from build123d import *

# Parameters (mm, degrees)
F1_DEPTH       = 3
F2_DEPTH       = 5.8
F3_D           = 3.3
F3_CSINK_D     = 6.72
F3_CSINK_ANGLE = 90


with BuildPart() as f1:
    # F0 (on Top) → F1 (new body)
    with BuildSketch(Plane.XY):
        with BuildLine():
            ThreePointArc((-3, 0), (0, 3), (3, 0))
            Line((3, 0), (45, 0))
            Line((45, 0), (45, 15))
            Line((45, 15), (-45, 15))
            Line((-45, 15), (-45, 0))
            Line((-45, 0), (-3, 0))
        make_face()
        with BuildLine():
            Line((45, 0), (3, 0))
            ThreePointArc((3, 0), (0, -3), (-3, 0))
            Line((-3, 0), (-45, 0))
            Line((-45, 0), (-45, -15))
            Line((-45, -15), (45, -15))
            Line((45, -15), (45, 0))
        make_face()
    extrude(amount=F1_DEPTH)

    # F0 (on Top) → F2 (join)
    with BuildSketch(Plane.XY):
        with BuildLine():
            Line((-3, 0), (3, 0))
            ThreePointArc((3, 0), (0, 3), (-3, 0))
        make_face()
        with BuildLine():
            ThreePointArc((-3, 0), (0, -3), (3, 0))
            Line((3, 0), (-3, 0))
        make_face()
    extrude(amount=F2_DEPTH)

    # F3 (through all)
    with Locations(Plane(origin=(0, 0, 0), x_dir=(1, 0, 0), z_dir=(0, 0, -1))):
        with Locations((-37, 0), (37, 0)):
            CounterSinkHole(F3_D / 2, F3_CSINK_D / 2, counter_sink_angle=F3_CSINK_ANGLE)


solid = f1.part
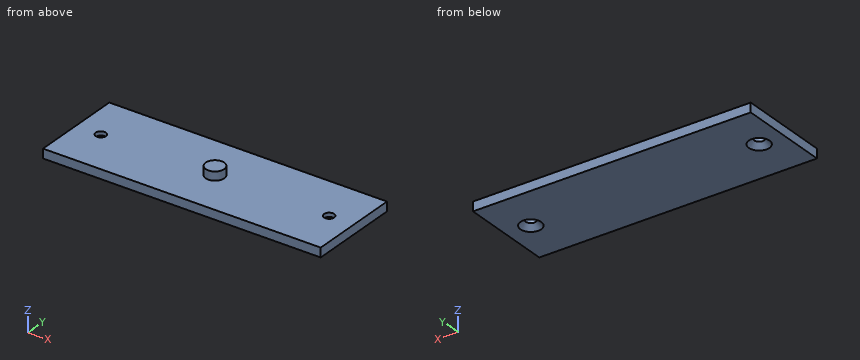
Design review of the part built by this model. Coordinates are the model's own, in mm. Round coordinates to 2 decimals unless told otherwise and drop trailing zeros. Write each loop counter-clockwise with the first axis right and the second up, starting at its lowest first coordinate (ties: lowest second). Pieces come first, ordered by that corner, then holes. Notation, with made-up numbers: (47.25, 72.25) - (65.25, 72.25) arc R6 cw to (65.25, 79.25) - close; hole circle Ø7 at (14, 64.5). An arc over 180 degrees is marked (long way). Use a Markdown table: item, result. Add a question column.
1. We need section B-B (x = 37). State the section outline as (y, z) points, then the cut area to 3 significant figures.
2. We need section D-D (z = 4.55). State the section outline as (x, y) points, then the cut area to 3 significant figures.
3. Clearance check with a flat-ended pin moving along its axis: pin 1 (15 mm diameter, centred on x = -20.5, y = 1.5, fed in from +Z). State where the tip first meets the part, or that it passes through.
4. We need section A-A (y = 0). State the section outline as (x, z) points, then the cut area to 3 significant figures.
5. We need section C-C (x = 0). State the section outline as (y, z) points.
6. Wall thickness on probe 1 along Y at (x, z) = (37, 2.4); probe 2 along Z at (x, y) = (-22.5, 5.75); probe 3 along X at (y, z) = (2.5, 5.15): over which ranges is each line inside the solid? List them lowest first.
Output:
| question | item | result |
|---|---|---|
| 1 | outline | (-15, 0) - (-3.36, 0) - (-1.65, 1.71) - (-1.65, 3) - (-15, 3) - close; (1.65, 1.71) - (3.36, 0) - (15, 0) - (15, 3) - (1.65, 3) - close |
| 1 | area | 77.2 mm2 |
| 2 | outline | circle Ø6 at (0, 0) |
| 2 | area | 28.3 mm2 |
| 3 | pin 1 | stops at z = 3 |
| 4 | outline | (-45, 0) - (-40.36, 0) - (-38.65, 1.71) - (-38.65, 3) - (-45, 3) - close; (-35.35, 1.71) - (-33.64, 0) - (33.64, 0) - (35.35, 1.71) - (35.35, 3) - (3, 3) - (3, 5.8) - (-3, 5.8) - (-3, 3) - (-35.35, 3) - close; (38.65, 1.71) - (40.36, 0) - (45, 0) - (45, 3) - (38.65, 3) - close |
| 4 | area | 261 mm2 |
| 5 | outline | (-15, 0) - (15, 0) - (15, 3) - (3, 3) - (3, 5.8) - (-3, 5.8) - (-3, 3) - (-15, 3) - close |
| 6 | probe 1 | y = -15 to -1.65, 1.65 to 15 |
| 6 | probe 2 | z = 0 to 3 |
| 6 | probe 3 | x = -1.66 to 1.66 |
